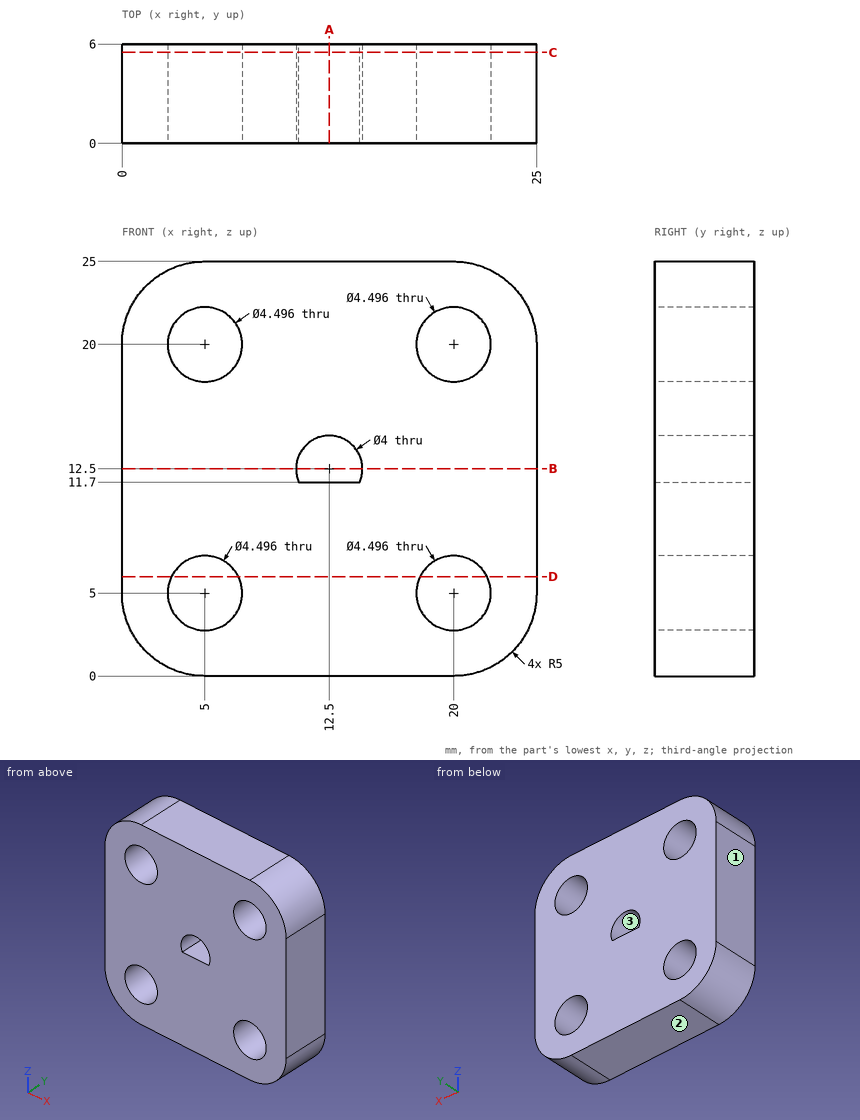
Check sheet for the drawn part. Datum: minimum x, y, z corner. Units: mm. Round coordinates to 2 decimals unless told otherwise and drop trailing zeros. Loops run counter-clockwise (first coordinate to the right, second up) from the corner with the lowest first, then second, coordinate; pieces in that order, holes last. Notation, with made-up numbers: (33, 29) - (54, 29) arc R18 ccw to (54, 42) - close; hole circle Ø4 at (8.25, 11.5). An arc over 180 degrees is marked (long way). Answer as a JSON object with one key per item and string values. Group by question number.
Q1. Sectioned sample at C-C, the plane y = 5.5. Enter the section's corners in (x, z).
Q2. Sectioned sample at B-B, the plane z = 12.5. Enter the section's corners in (x, y).
Q3. Gauge pin test, flat ends, axial feed: P1, Ø4, axis at x = 20, z = 20, coming from the -Y side; P2, Ø3, axis at y = 3.5, z = 12, coming from the -X side; P3, Ø1, axis at y = 5, z = 21.5, coming from the -X side; P4, Ø1.5, axis at y = 1.5, z = 22.5, coming from the -X side. Record the tip position at first contact, or that the pin passes through.
Q4. Mould release check, pull along X, two halves, no side actions. Record for the marked faces 1, 2 and 3: released by +X, released by -X, zero draft, split by the parting line, or undercut.
Q5. Scan lines: line 1 along X through (y, z) = (1.85, 20); line 2 along X through (y, z) = (1.05, 21). Record each from-to range of solid material in increasing order. Write a range as [from, to].
Q6. Sectioned sample at A-A, the plane x = 12.5. Enter the section's corners in (y, z), plus the area to 3 significant figures.
Q7. Sectioned sample at D-D, the plane z = 6. Enter the section's corners in (x, y), plus the area to 3 significant figures.
Solution:
{
 "1": {"outline": "(0, 5) arc R5 ccw to (5, 0) - (20, 0) arc R5 ccw to (25, 5) - (25, 20) arc R5 ccw to (20, 25) - (5, 25) arc R5 ccw to (0, 20) - close; hole circle Ø4.5 at (5, 5); hole circle Ø4.5 at (5, 20); hole (10.67, 11.7) - (14.33, 11.7) arc R2 ccw (long way) to start; hole circle Ø4.5 at (20, 5); hole circle Ø4.5 at (20, 20)"},
 "2": {"outline": "(0, 0) - (10.5, 0) - (10.5, 6) - (0, 6) - close; (14.5, 0) - (25, 0) - (25, 6) - (14.5, 6) - close"},
 "3": {"P1": "passes through", "P2": "stops at x = 0", "P3": "stops at x = 0.1", "P4": "stops at x = 0.32"},
 "4": {"face 1": "released by -X", "face 2": "zero draft", "face 3": "undercut"},
 "5": {"line 1": "x = [0, 2.75], [7.25, 17.75], [22.25, 25]", "line 2": "x = [0.1, 2.99], [7.01, 17.99], [22.01, 24.9]"},
 "6": {"outline": "(0, 0) - (6, 0) - (6, 11.7) - (0, 11.7) - close; (0, 14.5) - (6, 14.5) - (6, 25) - (0, 25) - close", "area": "133 mm²"},
 "7": {"outline": "(0, 0) - (2.99, 0) - (2.99, 6) - (0, 6) - close; (7.01, 0) - (17.99, 0) - (17.99, 6) - (7.01, 6) - close; (22.01, 0) - (25, 0) - (25, 6) - (22.01, 6) - close", "area": "102 mm²"}
}
